```python
from build123d import *

# Parameters (mm, degrees)
BOSS_EXTRUDE1_DEPTH                      = 50.8
CBORE_FOR_M12_HEX_HEAD_BOLT1_D           = 13.5
CBORE_FOR_M12_HEX_HEAD_BOLT1_CBORE_D     = 23.78
CBORE_FOR_M12_HEX_HEAD_BOLT1_CBORE_DEPTH = 7.95
BOSS_EXTRUDE2_DEPTH                      = 12.7
FILLET1_R                                = 12.7


with BuildPart() as part:
    # Sketch1 → Boss-Extrude1 (new, symmetric)
    with BuildSketch(Plane.XY):
        Polygon((0, 0), (101.6, 0), (101.6, 25.4), (101.6, 95.25), (76.2, 95.25), (76.2, 25.4), (0, 25.4), align=None)
    extrude(amount=BOSS_EXTRUDE1_DEPTH, both=True)

    # CBORE for M12 Hex Head Bolt1 (through all)
    with Locations(Plane.ZY.offset(-76.2)):
        with Locations((0, 60.325)):
            CounterBoreHole(CBORE_FOR_M12_HEX_HEAD_BOLT1_D / 2, CBORE_FOR_M12_HEX_HEAD_BOLT1_CBORE_D / 2, CBORE_FOR_M12_HEX_HEAD_BOLT1_CBORE_DEPTH)

    # Sketch5 → Boss-Extrude2 (add)
    with BuildSketch(Plane(origin=(0, 0, -50.8), x_dir=(-1, 0, 0), z_dir=(0, 0, -1))):
        Polygon((-76.2, 95.25), (0, 25.4), (-76.2, 25.4), align=None)
    boss_extrude2 = extrude(amount=-BOSS_EXTRUDE2_DEPTH)

    # Mirror1: Boss-Extrude2 across plane
    add(boss_extrude2.mirror(Plane.XY))

    # Fillet1
    fillet1_edges = [part.edges().sort_by_distance(p)[0] for p in [
        (38.1, 25.4, -38.1),
        (76.2, 25.4, 0),
        (38.1, 25.4, 38.1),
    ]]
    fillet(fillet1_edges, radius=FILLET1_R)


solid = part.part
```
For this review, take the finished solid that the model builds, in its own axes (mm). A direction names the side the tool comes from. Coordinates: 2 decimals unless noted, no trailing zeros. Loops run counter-clockwise (first coordinate to the right, second up) from the corner with the lowest first, then second, coordinate; pieces in that order, holes last. Notation, with made-up numbers: (-34, 26) - (-20, 26) arc R4 ccw to (-20, 32) - close; hole circle Ø7 at (62, 14.5). An arc over 180 degrees is marked (long way). Use one line per item in the form item = value. Start each with the question number.
1) For pin 1 (19 mm diameter, centred on y = 60.325, z = 0, fed in from -X); pin 2 (1.5 mm diameter, centred on y = 29.5, z = -39, fed in from -X), all flat-tipped, find the tip position at first contact; note any pin that passes through.
2) Take a section at A-A (z = 23). State the section outline as (x, y) points.
3) Take a section at D-D (y = 51.5). State the section outline as (x, z) points, plus the area to 3 significant figures.
4) Take a section at B-B (z = 0). State the section outline as (x, y) points (3 decimals).
5) For faces 1 (the face through (38.63, 29.22, 34.48)), 2 (the face through (80.12, 48.72, -2.58)), 3 (the face through (0, 13, 1)), list the 3-axis set-ups (+Z, -Z, +X, -X, +Y, -Y) from which the entire face can be reached by the end or side of a thin tool; tool diameter is ignored.
6) Draft analysis for pull direction Y (two halves, no side actions). For faces 4 (the face through (89, 95.25, 1)), 5 (the face through (58, 54, 38.1)), 6 (the face through (84.15, 55, 5)), state which applies: released by +Y, released by -Y, zero draft, split by the parting line, or undercut.
7) Take a section at C-C (x = 49.5). State the section outline as (y, z) points (3 decimals), plus the area to 3 significant figures.
8) To check wall thickness, follow probe 1 along Z at (x, y) = (42.5, 39.5); probe 2 along Y at (x, z) = (88, 0) (3 decimals); probe 3 along Y at (x, z) = (27.5, -9.5). State the ranges of each line that lie inside material, in increasing order. Write a range as from..to.
From the geometry:
q1.pin_1 = 84.15
q1.pin_2 = 3.65
q2.outline = (0, 0) - (101.6, 0) - (101.6, 95.25) - (76.2, 95.25) - (76.2, 38.1) arc R12.7 cw to (63.5, 25.4) - (0, 25.4) - close
q3.outline = (28.47, -50.8) - (101.6, -50.8) - (101.6, 50.8) - (28.47, 50.8) - (28.47, 38.1) - (76.2, 38.1) - (76.2, 7.97) - (84.15, 7.97) - (84.15, -7.97) - (76.2, -7.97) - (76.2, -38.1) - (28.47, -38.1) - close
q3.area = 3,670 mm2
q4.outline = (0, 0) - (101.6, 0) - (101.6, 53.575) - (84.15, 53.575) - (84.15, 48.435) - (76.2, 48.435) - (76.2, 38.1) arc R12.7 cw to (63.5, 25.4) - (0, 25.4) - close; (76.2, 72.215) - (84.15, 72.215) - (84.15, 67.075) - (101.6, 67.075) - (101.6, 95.25) - (76.2, 95.25) - close
q5.face_1 = -X, +Y
q5.face_2 = -X
q5.face_3 = +Z, -Z, -X, +Y, -Y
q6.face_4 = released by +Y
q6.face_5 = zero draft
q6.face_6 = undercut
q7.outline = (0, -50.8) - (70.775, -50.8) - (70.775, -38.1) - (38.1, -38.1) arc R12.7 cw to (25.4, -25.4) - (25.4, 25.4) arc R12.7 cw to (38.1, 38.1) - (70.775, 38.1) - (70.775, 50.8) - (0, 50.8) - close
q7.area = 3,800 mm2
q8.probe_1 = -50.8..-38.1, 38.1..50.8
q8.probe_2 = 0..53.575, 67.075..95.25
q8.probe_3 = 0..25.4
